Here's how the part is built. I have some questions about the finished solid (model axes, mm). Face numbers are marked on the shaded views. Round coordinates to 2 decimals unless told otherwise and drop trailing zeros. Order: outer loops, then holes, each group sorted by start corner. A loop starts at its lowest first (then second) coordinate and runs counter-clockwise, first axis right, second up. Notation, with made-up numbers: M 20,-35 L 58,-35 A27 ccw 58,-17 Z; hole C 48,38 d2. An arc over 180 degrees is marked long. Use one line per item in the form item = value. Start each with the question number.
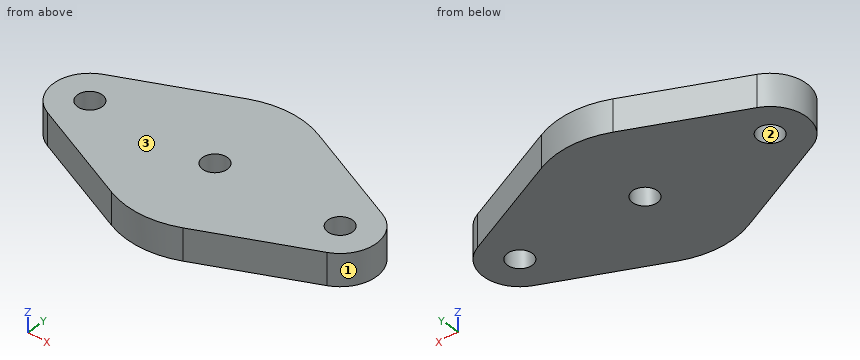
```python
from build123d import *

# Parameters (mm, degrees)
F0_R     = 13.9065
F0_R_2   = 9.906
F1_DEPTH = 25.4


with BuildPart() as f1:
    # F0 (on Top) → F1 (new body)
    with BuildSketch(Plane.XY):
        with BuildLine():
            Line((70.7064372, 0), (64.77, 0))
            ThreePointArc((64.77, 0), (0, -64.77), (-64.77, 0))
            Line((-64.77, 0), (-70.7064372, 0))
            ThreePointArc((-70.7064372, 0), (-59.3851891605, -38.3770708873), (-29.0468761129, -64.4645580889))
            ThreePointArc((-29.0468761129, -64.4645580889), (0, -70.7064372), (29.0468761129, -64.4645580889))
            ThreePointArc((29.0468761129, -64.4645580889), (59.3851891605, -38.3770708873), (70.7064372, 0))
        make_face()
        with BuildLine():
            ThreePointArc((-64.77, 0), (0, 64.77), (64.77, 0))
            Line((64.77, 0), (70.7064372, 0))
            ThreePointArc((70.7064372, 0), (59.3851891605, 38.3770708873), (29.0468761129, 64.4645580889))
            ThreePointArc((29.0468761129, 64.4645580889), (0, 70.7064372), (-29.0468761129, 64.4645580889))
            ThreePointArc((-29.0468761129, 64.4645580889), (-59.3851891605, 38.3770708873), (-70.7064372, 0))
            Line((-70.7064372, 0), (-64.77, 0))
        make_face()
        with BuildLine():
            Line((72.631808, 0), (70.7064372, 0))
            ThreePointArc((70.7064372, 0), (59.3851891605, -38.3770708873), (29.0468761129, -64.4645580889))
            Line((29.0468761129, -64.4645580889), (113.5004084714, -26.410914902))
            ThreePointArc((113.5004084714, -26.410914902), (85.8770417817, -24.3299143569), (72.631808, 0))
        make_face()
        with BuildLine():
            ThreePointArc((29.0468761129, 64.4645580889), (59.3851891605, 38.3770708873), (70.7064372, 0))
            Line((70.7064372, 0), (72.631808, 0))
            ThreePointArc((72.631808, 0), (85.8770417817, 24.3299143569), (113.5004084714, 26.410914902))
            Line((113.5004084714, 26.410914902), (29.0468761129, 64.4645580889))
        make_face()
        with BuildLine():
            Line((-72.631808, 0), (-70.7064372, 0))
            ThreePointArc((-70.7064372, 0), (-59.3851891605, 38.3770708873), (-29.0468761129, 64.4645580889))
            Line((-29.0468761129, 64.4645580889), (-113.5004084714, 26.410914902))
            ThreePointArc((-113.5004084714, 26.410914902), (-85.8770417817, 24.3299143569), (-72.631808, 0))
        make_face()
        with BuildLine():
            ThreePointArc((-29.0468761129, -64.4645580889), (-59.3851891605, -38.3770708873), (-70.7064372, 0))
            Line((-70.7064372, 0), (-72.631808, 0))
            ThreePointArc((-72.631808, 0), (-85.8770417817, -24.3299143569), (-113.5004084714, -26.410914902))
            Line((-113.5004084714, -26.410914902), (-29.0468761129, -64.4645580889))
        make_face()
        with BuildLine():
            ThreePointArc((113.5004084714, 26.410914902), (85.8770417817, 24.3299143569), (72.631808, 0))
            ThreePointArc((72.631808, 0), (85.8770417817, -24.3299143569), (113.5004084714, -26.410914902))
            ThreePointArc((113.5004084714, -26.410914902), (125.9299143569, -15.7229582183), (130.568192, 0))
            ThreePointArc((130.568192, 0), (125.9299143569, 15.7229582183), (113.5004084714, 26.410914902))
        make_face()
        with BuildLine():
            ThreePointArc((115.5065, 0), (101.6, -13.9065), (87.6935, 0))
            ThreePointArc((87.6935, 0), (101.6, 13.9065), (115.5065, 0))
        make_face(mode=Mode.SUBTRACT)
        with BuildLine():
            ThreePointArc((-113.5004084714, -26.410914902), (-85.8770417817, -24.3299143569), (-72.631808, 0))
            ThreePointArc((-72.631808, 0), (-85.8770417817, 24.3299143569), (-113.5004084714, 26.410914902))
            ThreePointArc((-113.5004084714, 26.410914902), (-130.568192, 0), (-113.5004084714, -26.410914902))
        make_face()
        with Locations((-101.6, 0)):
            Circle(F0_R, mode=Mode.SUBTRACT)
        with BuildLine():
            ThreePointArc((-64.77, 0), (0, -64.77), (64.77, 0))
            Line((64.77, 0), (9.906, 0))
            ThreePointArc((9.906, 0), (0, -9.906), (-9.906, 0))
            Line((-9.906, 0), (-64.77, 0))
        make_face()
        with BuildLine():
            Line((9.906, 0), (64.77, 0))
            ThreePointArc((64.77, 0), (0, 64.77), (-64.77, 0))
            Line((-64.77, 0), (-9.906, 0))
            ThreePointArc((-9.906, 0), (0, 9.906), (9.906, 0))
        make_face()
        with BuildLine():
            ThreePointArc((115.5065, 0), (101.6, 13.9065), (87.6935, 0))
            ThreePointArc((87.6935, 0), (101.6, -13.9065), (115.5065, 0))
        make_face()
        with BuildLine():
            ThreePointArc((111.506, 0), (101.6, -9.906), (91.694, 0))
            ThreePointArc((91.694, 0), (101.6, 9.906), (111.506, 0))
        make_face(mode=Mode.SUBTRACT)
        with Locations((-101.6, 0)):
            Circle(F0_R)
        with Locations((-101.6, 0)):
            Circle(F0_R_2, mode=Mode.SUBTRACT)
    extrude(amount=F1_DEPTH)


solid = f1.part
```
1) If I drill on line 1 (Y direction, x = 0, z = 8); line 2 (Y direction, x = 101.6, z = 12.25); line 3 (X direction, y = -8.5, z = 22.75), over which ranges is the centre line in solid material (lowest first)?
2) If we section it at B-B on z = 10: Write out the boundary of the cut face in (x, y).
3) Will these pins go through, and if not, where does the flat tip stop? pin 1 Ø10 at (y, z) = (-4, 3.5) entering from -X; pin 2 Ø3 at (x, z) = (-11, 12.5) entering from -Y; pin 3 Ø5 at (x, z) = (62, 18.5) entering from +Y.
4) If we mould it in two halves opening along X, with no side actions, what happens to the marked faces 1, 2 and 3? For each: +X half, -X half, draft (parallel to the pull), parting line (faces both ways), or undercut.
5) If we section it at D-D on x = 101.6: Write out the boundary of the cut face in (y, z).
6) If we section it at C-C on y = 0: Write out the boundary of the cut face in (x, z).
7) If we section it at A-A on x = 0: Write out the boundary of the cut face in (y, z), then the cut area to 3 significant figures.
Completed:
q1.line_1 = -70.71 to -9.91, 9.91 to 70.71
q1.line_2 = -31.77 to -9.91, 9.91 to 31.77
q1.line_3 = -129.29 to -106.69, -96.51 to -5.09, 5.09 to 96.51, 106.69 to 129.29
q2.outline = M -113.5,-26.41 L -29.05,-64.46 A70.71 ccw 29.05,-64.46 L 113.5,-26.41 A28.97 ccw 113.5,26.41 L 29.05,64.46 A70.71 ccw -29.05,64.46 L -113.5,26.41 A28.97 ccw Z; hole C -101.6,0 d19.81; hole C 0,0 d19.81; hole C 101.6,0 d19.81
q3.pin_1 = -130.57
q3.pin_2 = -70.07
q3.pin_3 = 50.74
q4.face_1 = +X half
q4.face_2 = undercut
q4.face_3 = draft
q5.outline = M -31.77,0 L -9.91,0 L -9.91,25.4 L -31.77,25.4 Z; M 9.91,0 L 31.77,0 L 31.77,25.4 L 9.91,25.4 Z
q6.outline = M -130.57,0 L -111.51,0 L -111.51,25.4 L -130.57,25.4 Z; M -91.69,0 L -9.91,0 L -9.91,25.4 L -91.69,25.4 Z; M 9.91,0 L 91.69,0 L 91.69,25.4 L 9.91,25.4 Z; M 111.51,0 L 130.57,0 L 130.57,25.4 L 111.51,25.4 Z
q7.outline = M -70.71,0 L -9.91,0 L -9.91,25.4 L -70.71,25.4 Z; M 9.91,0 L 70.71,0 L 70.71,25.4 L 9.91,25.4 Z
q7.area = 3,090 mm²
